Here's how the part is built. I have some questions about the finished solid (model axes, mm). Face numbers are marked on the shaded views. A direction names the side the tool comes from. Coordinates: 2 decimals unless noted, no trailing zeros. Loops run counter-clockwise (first coordinate to the right, second up) from the corner with the lowest first, then second, coordinate; pieces in that order, holes last. Notation, with made-up numbers: (73, -5.5) -> (113, -5.5) arc R27 ccw to (113, 24.5) -> close; hole circle Ø11 at (-25.75, -13.5). An arc over 180 degrees is marked (long way). Answer as a JSON object with one key per item and string values. Group by question number.
1) I need wall thicknesses on probe 1 along Y at (x, z) = (8.75, 1.6); probe 2 along Y at (x, z) = (-8.75, -0.15); probe 3 along X at (y, z) = (1.5, 0.9). Which ranges of each line are inside material? Lowest first, please. Write a range as [from, to].
2) I want a section at B-B (x = 8.75). Write out the boundary of the cut face in (y, z).
3) I'm going to push flat-ended pins straight in: pin 1 (3 mm diameter, centred on x = 1.5, y = 1.5, fed in from -Z); pin 2 (3 mm diameter, centred on x = -8.5, y = -0.5, fed in from +Z); pin 3 (1.1 mm diameter, centred on x = 9.5, y = -0.5, fed in from +Z); pin 4 (1 mm diameter, centred on y = 2.5, z = 1, fed in from -X). Where does each tip first touch, or does it pass through?
4) I want a section at A-A (z = -0.3). Write out the boundary of the cut face in (x, y).
5) If we mould it in two halves opening along Y, with no side actions, what happens to the marked faces 4, 5, 6 and 7? For each: +Y half, -Y half, draft (parallel to the pull), parting line (faces both ways), or undercut.
6) I want a section at C-C (z = 1.35). Write out the boundary of the cut face in (x, y), then the cut area to 3 significant figures.
7) Which directions (+Z, -Z, +X, -X, +Y, -Y) give clear straight access to the entire face, cutting with the end or side of a thin tool? Please do the marked faces 1, 2 and 3.
8) I want a section at D-D (y = -1.5). Write out the boundary of the cut face in (x, z).
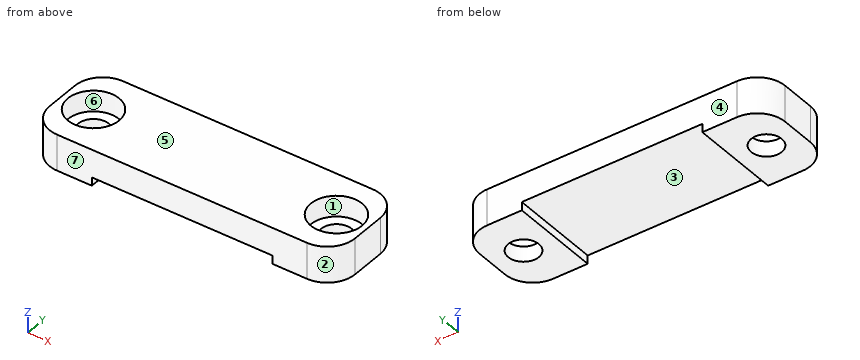
```python
from build123d import *

# Parameters (mm, degrees)
F0_W           = 22
F0_H           = 6.5
F1_DEPTH       = 2
F2_W           = 4.5
F2_H           = 6.5
F3_DEPTH       = 0.6
F6_D           = 2.2
F6_CBORE_D     = 3.7
F6_CBORE_DEPTH = 1.5
F7_R           = 2


with BuildPart() as f1:
    # F0 (on Top) → F1 (new body)
    with BuildSketch(Plane.XY):
        Rectangle(F0_W, F0_H)
    extrude(amount=F1_DEPTH)

    # F2 (on Top) → F3 (join)
    with BuildSketch(Plane.XY):
        with Locations((-8.75, 0)):
            Rectangle(F2_W, F2_H)
        with Locations((8.75, 0)):
            Rectangle(F2_W, F2_H)
    extrude(amount=-F3_DEPTH)

    # F6 (through all)
    with Locations(Plane.XY.offset(2)):
        with Locations((-8.75, 0), (8.75, 0)):
            CounterBoreHole(F6_D / 2, F6_CBORE_D / 2, F6_CBORE_DEPTH)

    # F7
    f7_edges = [f1.edges().sort_by_distance(p)[0] for p in [
        (-11, -3.25, 0.7),
        (-11, 3.25, 0.7),
        (11, -3.25, 0.7),
        (11, 3.25, 0.7),
    ]]
    fillet(f7_edges, radius=F7_R)


solid = f1.part
```
Determined:
{
 "1": {"probe 1": "[-3.25, -1.85], [1.85, 3.25]", "probe 2": "[-3.25, -1.1], [1.1, 3.25]", "probe 3": "[-10.98, -9.83], [-7.67, 7.67], [9.83, 10.98]"},
 "2": {"outline": "(-3.25, -0.6) -> (-1.1, -0.6) -> (-1.1, 0.5) -> (-1.85, 0.5) -> (-1.85, 2) -> (-3.25, 2) -> close; (1.1, -0.6) -> (3.25, -0.6) -> (3.25, 2) -> (1.85, 2) -> (1.85, 0.5) -> (1.1, 0.5) -> close"},
 "3": {"pin 1": "z = 0", "pin 2": "z = 2", "pin 3": "z = 0.5", "pin 4": "x = -10.85"},
 "4": {"outline": "(-11, -1.25) arc R2 ccw to (-9, -3.25) -> (-6.5, -3.25) -> (-6.5, 3.25) -> (-9, 3.25) arc R2 ccw to (-11, 1.25) -> close; (6.5, -3.25) -> (9, -3.25) arc R2 ccw to (11, -1.25) -> (11, 1.25) arc R2 ccw to (9, 3.25) -> (6.5, 3.25) -> close; hole circle Ø2.2 at (-8.75, 0); hole circle Ø2.2 at (8.75, 0)"},
 "5": {"face 4": "+Y half", "face 5": "draft", "face 6": "undercut", "face 7": "-Y half"},
 "6": {"outline": "(-11, -1.25) arc R2 ccw to (-9, -3.25) -> (9, -3.25) arc R2 ccw to (11, -1.25) -> (11, 1.25) arc R2 ccw to (9, 3.25) -> (-9, 3.25) arc R2 ccw to (-11, 1.25) -> close; hole circle Ø3.7 at (-8.75, 0); hole circle Ø3.7 at (8.75, 0)", "area": "118 mm^2"},
 "7": {"face 1": "+Z", "face 2": "+Z, -Z, +X, -Y", "face 3": "-Z, +Y, -Y"},
 "8": {"outline": "(-10.98, -0.6) -> (-6.5, -0.6) -> (-6.5, 0) -> (6.5, 0) -> (6.5, -0.6) -> (10.98, -0.6) -> (10.98, 2) -> (9.83, 2) -> (9.83, 0.5) -> (7.67, 0.5) -> (7.67, 2) -> (-7.67, 2) -> (-7.67, 0.5) -> (-9.83, 0.5) -> (-9.83, 2) -> (-10.98, 2) -> close"}
}
